from build123d import *

# Parameters (mm, degrees)
BOSS_EXTRUDE1_START      = -8
SKETCH2_W                = 26
SKETCH2_H                = 36
SKETCH2_W_2              = 18
SKETCH2_H_2              = 12
BOSS_EXTRUDE1_DEPTH      = 5
BOSS_EXTRUDE2_START      = -3
SKETCH2_7_W              = 17
SKETCH2_7_H              = 5
BOSS_EXTRUDE2_DEPTH      = 19.1
BOSS_EXTRUDE3_START      = 11.1
SKETCH2_14_W             = 17
SKETCH2_14_H             = 18.5
BOSS_EXTRUDE3_DEPTH      = 5
M3_CLEARANCE_HOLE1_D     = 3.2
M3_CLEARANCE_HOLE1_DEPTH = 5
M3_CLEARANCE_HOLE1_TIP   = 0.96137699
FILLET1_START            = -8.5
FILLET1_DEPTH            = 17
FILLET1_2_DEPTH          = 1.500148193
FILLET1_START_2          = 6.999851807
FILLET1_3_DEPTH          = 1.500148193
FILLET1_START_3          = 5.377704746
FILLET1_4_DEPTH          = 5.722295254
FILLET1_START_4          = 5.601514307
FILLET1_5_DEPTH          = 5.498485693
FILLET1_START_5          = 4.22249738
FILLET1_6_DEPTH          = 5.871975237
FILLET1_START_6          = -6.999851807
FILLET1_7_DEPTH          = 13.999703614
FILLET3_R                = 1


with BuildPart() as part:
    # Sketch2 → Boss-Extrude1 (new body)
    with BuildSketch(Plane(origin=(0, 0, 0), x_dir=(0, 0, -1), z_dir=(1, 0, 0)).offset(BOSS_EXTRUDE1_START)):
        with Locations((0, 9.5)):
            Rectangle(SKETCH2_W, SKETCH2_H)
        with Locations((0, 13.5)):
            Rectangle(SKETCH2_W_2, SKETCH2_H_2, mode=Mode.SUBTRACT)
    extrude(amount=BOSS_EXTRUDE1_DEPTH)

    # Sketch2<7> → Boss-Extrude2 (add)
    with BuildSketch(Plane(origin=(0, 0, 0), x_dir=(0, 0, -1), z_dir=(1, 0, 0)).offset(BOSS_EXTRUDE2_START)):
        with Locations((0, 25)):
            Rectangle(SKETCH2_7_W, SKETCH2_7_H)
    extrude(amount=BOSS_EXTRUDE2_DEPTH)

    # Sketch2<14> → Boss-Extrude3 (add)
    with BuildSketch(Plane(origin=(0, 0, 0), x_dir=(0, 0, -1), z_dir=(1, 0, 0)).offset(BOSS_EXTRUDE3_START)):
        with Locations((0, 36.75)):
            Rectangle(SKETCH2_14_W, SKETCH2_14_H)
        with BuildLine():
            Line((3, 28), (-3, 28))
            ThreePointArc((-3, 28), (-7, 32), (-3, 36))
            Line((-3, 36), (3, 36))
            ThreePointArc((3, 36), (7, 32), (3, 28))
        make_face(mode=Mode.SUBTRACT)
    extrude(amount=BOSS_EXTRUDE3_DEPTH)

    # M3 Clearance Hole1
    with Locations(Plane.ZY.offset(-11.1)):
        with Locations((5, 41), (-5, 41)):
            Hole(M3_CLEARANCE_HOLE1_D / 2, depth=M3_CLEARANCE_HOLE1_DEPTH)
            with Locations((0, 0, -(M3_CLEARANCE_HOLE1_DEPTH + M3_CLEARANCE_HOLE1_TIP / 2))):  # 118° drill point
                Cone(0, M3_CLEARANCE_HOLE1_D / 2, M3_CLEARANCE_HOLE1_TIP, mode=Mode.SUBTRACT)

    # Fillet1: read off the stored shape, not the designer's step
    # Fillet1 outline → Fillet1 (add)
    with BuildSketch(Plane.XY.offset(FILLET1_START)):
        with BuildLine():
            Line((11.1, 28), (4.222498999, 28))
            ThreePointArc((4.222498999, 28), (2.68113883, 27.625791171), (1.1, 27.5))
            Line((1.1, 27.5), (11.1, 27.5))
            Line((11.1, 27.5), (11.1, 28))
        make_face()
        with BuildLine():
            ThreePointArc((11.1, 37.5), (11.071674876, 36.747869581), (10.986859967, 36))
            Line((10.986859967, 36), (11.1, 36))
            Line((11.1, 36), (11.1, 37.5))
        make_face()
    extrude(amount=FILLET1_DEPTH)

    # Fillet1 2 outline → Fillet1 2 (add)
    with BuildSketch(Plane.XY.offset(FILLET1_START)):
        with BuildLine():
            ThreePointArc((10.986859967, 36), (8.736154476, 31.04328684), (4.222498999, 28))
            Line((4.222498999, 28), (11.1, 28))
            Line((11.1, 28), (11.1, 36))
            Line((11.1, 36), (10.986859967, 36))
        make_face()
    extrude(amount=FILLET1_2_DEPTH)

    # Fillet1 3 outline → Fillet1 3 (add)
    with BuildSketch(Plane.XY.offset(FILLET1_START_2)):
        with BuildLine():
            ThreePointArc((10.986859967, 36), (8.736154476, 31.04328684), (4.222498999, 28))
            Line((4.222498999, 28), (11.1, 28))
            Line((11.1, 28), (11.1, 36))
            Line((11.1, 36), (10.986859967, 36))
        make_face()
    extrude(amount=FILLET1_3_DEPTH)

    # Fillet1 4 outline → Fillet1 4 (cut)
    with BuildSketch(Plane.YZ.offset(FILLET1_START_3)):
        with BuildLine():
            Line((31.965568589, 6.999851807), (32.034431411, 6.999851807))
            ThreePointArc((32.034431411, 6.999851807), (32, 7), (31.965568589, 6.999851807))
        make_face()
        with BuildLine():
            ThreePointArc((31.965568589, -6.999851807), (32, -7), (32.034431411, -6.999851807))
            Line((32.034431411, -6.999851807), (31.965568589, -6.999851807))
        make_face()
    extrude(amount=FILLET1_4_DEPTH, mode=Mode.SUBTRACT)

    # Fillet1 5 outline → Fillet1 5 (add)
    with BuildSketch(Plane.YZ.offset(FILLET1_START_4)):
        with BuildLine():
            ThreePointArc((32.034431411, 6.999851807), (34.840574382, 5.816227473), (36, 3))
            Line((36, 3), (36, 6.999851807))
            Line((36, 6.999851807), (32.034431411, 6.999851807))
        make_face()
        with BuildLine():
            Line((36, -6.999851807), (36, -3))
            ThreePointArc((36, -3), (34.840574382, -5.816227473), (32.034431411, -6.999851807))
            Line((32.034431411, -6.999851807), (36, -6.999851807))
        make_face()
        with BuildLine():
            ThreePointArc((28, 3), (29.159425618, 5.816227473), (31.965568589, 6.999851807))
            Line((31.965568589, 6.999851807), (28, 6.999851807))
            Line((28, 6.999851807), (28, 3))
        make_face()
        with BuildLine():
            Line((28, -6.999851807), (31.965568589, -6.999851807))
            ThreePointArc((31.965568589, -6.999851807), (29.159425618, -5.816227473), (28, -3))
            Line((28, -3), (28, -6.999851807))
        make_face()
    extrude(amount=FILLET1_5_DEPTH)

    # Fillet1 6 outline → Fillet1 6 (add)
    with BuildSketch(Plane.YZ.offset(FILLET1_START_5)):
        with BuildLine():
            ThreePointArc((28, 3), (29.159425618, 5.816227473), (31.965568589, 6.999851807))
            Line((31.965568589, 6.999851807), (28, 6.999851807))
            Line((28, 6.999851807), (28, 3))
        make_face()
        with BuildLine():
            Line((28, -6.999851807), (31.965568589, -6.999851807))
            ThreePointArc((31.965568589, -6.999851807), (29.159425618, -5.816227473), (28, -3))
            Line((28, -3), (28, -6.999851807))
        make_face()
    extrude(amount=FILLET1_6_DEPTH)

    # Fillet1 7 outline → Fillet1 7 (cut)
    with BuildSketch(Plane.XY.offset(FILLET1_START_6)):
        with BuildLine():
            ThreePointArc((4.222497538, 27.99999952), (8.736153979, 31.043286253), (10.986859967, 36))
            ThreePointArc((10.986859967, 36), (11.049747147, 36.498734945), (11.087492178, 37))
            Line((11.087492178, 37), (3, 37))
            Line((3, 37), (3, 27.682159097))
            ThreePointArc((3, 27.682159097), (3.616272245, 27.821757701), (4.222497538, 27.99999952))
        make_face()
    extrude(amount=FILLET1_7_DEPTH, mode=Mode.SUBTRACT)

    # Fillet3
    fillet3_edges = [part.edges().sort_by_distance(p)[0] for p in [
        (6.55, 22.5, -8.5),
        (6.55, 22.5, 8.5),
        (13.6, 46, -8.5),
        (13.6, 46, 8.5),
    ]]
    fillet(fillet3_edges, radius=FILLET3_R)


solid = part.part
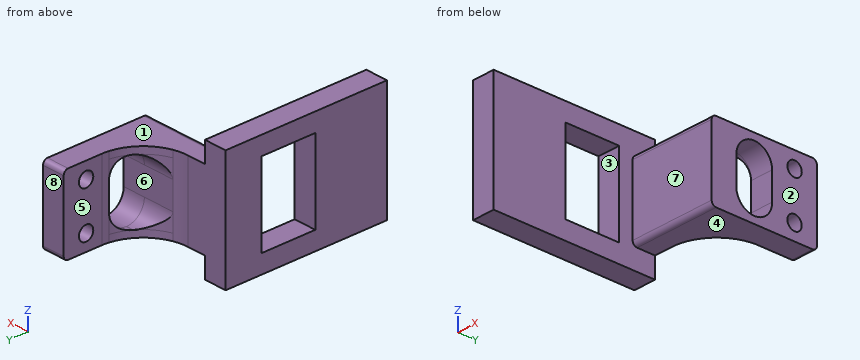
Geometry check sheet. Reference: the model listing, model coordinates, mm. Face numbers are marked on the shaded views. A direction names the side the tool comes from. Round coordinates to 2 decimals unless told otherwise and drop trailing zeros. Order: outer loops, then holes, each group sorted by start corner. A loop starts at its lowest first (then second) coordinate and runs counter-clockwise, first axis right, second up. Notation, with made-up numbers: M 69.25,-20 L 117.25,-20 A36 cw 117.25,15 Z; hole C 78.5,3 d2. An arc over 180 degrees is marked long. Write each question's results on one line, items separated by ' | '. Start each with the question number.
1. Cross-section at A-A on y = 41. Record the boundary of the cut face in (x, z).
2. Set-up check for the marked faces 5, 6, 7 and 8: record each of +Z, -Z, +X, -X, +Y, -Y from which the full face is reachable in a straight line by a thin tool's end or side.
3. Cross-section at D-D on y = 26. Record the boundary of the cut face in (x, z), plus the area to 3 significant figures.
4. Cross-section at C-C on z = 5. Record the boundary of the cut face in (x, y).
5. Go/stop test with flat-tipped pins: P1, Ø1.5, axis at x = 1.5, y = 26, coming from the +Z side; P2, Ø2.5, axis at y = 43.5, z = 3.5, coming from the -X side; P3, Ø6, axis at x = 1.5, z = 6.5, coming from the -Y side; P4, Ø1.5, axis at x = -1.5, y = 21.5, coming from the -Z side. Record where each tip stops, or that it passes through.
6. Cross-section at B-B on x = 12. Record the boundary of the cut face in (y, z).
7. Material ranges on L1, parallel to Z at x = 13.1, y = 41; L2, parallel to Y at x = -4.75, z = -1; L3, parallel to Y at x = 14.1, z = -5, recorded low to high. Write a range as from..to.
8. Draft check along Z on the marked faces 1, 2, 3 and 4. Enter one of: pulls with the +Z half, pulls with the -Z half, needs draft (parallel to the pull), parting line crosses it, or undercut.
Resolved:
1) outline: M 11.1,-8.5 L 16.1,-8.5 L 16.1,-6.6 L 11.1,-6.6 Z; M 11.1,-3.4 L 16.1,-3.4 L 16.1,3.4 L 11.1,3.4 Z; M 11.1,6.6 L 16.1,6.6 L 16.1,8.5 L 11.1,8.5 Z
2) face 5: +Z, -Z, -X, +Y | face 6: +X, -X | face 7: +Z, -Z, +X, -Y | face 8: +Z, -Z, +X, -X, +Y
3) outline: M -8,-13 L -3,-13 L -3,-8.5 L 16.1,-8.5 L 16.1,8.5 L -3,8.5 L -3,13 L -8,13 Z | area: 455 mm2
4) outline: M -8,-8.5 L -3,-8.5 L -3,7.5 L -8,7.5 Z; M -8,19.5 L -3,19.5 L -3,22.5 L 16.1,22.5 L 16.1,28.54 L 5.53,28.54 A10 cw 1.1,27.5 L -8,27.5 Z; M 10.89,35.46 L 16.1,35.46 L 16.1,39.4 L 11.1,39.4 L 11.1,37.5 A10 cw Z; M 11.1,42.6 L 16.1,42.6 L 16.1,46 L 11.1,46 Z
5) P1: z = 8.5 | P2: x = 11.1 | P3: y = 22.5 | P4: through
6) outline: M 22.5,-7.5 A1 ccw 23.5,-8.5 L 45,-8.5 A1 ccw 46,-7.5 L 46,7.5 A1 ccw 45,8.5 L 23.5,8.5 A1 ccw 22.5,7.5 Z; hole M 28,-3 A4 ccw 36,-3 L 36,3 A4 ccw 28,3 Z; hole C 41,-5 d3.2; hole C 41,5 d3.2
7) L1: -8.5..-6.6, -3.4..3.4, 6.6..8.5 | L2: -8.5..7.5, 19.5..27.5 | L3: 22.5..28.54, 35.46..39.4, 42.6..46
8) face 1: pulls with the +Z half | face 2: needs draft | face 3: undercut | face 4: pulls with the -Z half
